Here's the drawing with two shaded views (mm, measured from the low corner). I have some questions. A direction names the side the tool comes from. Give positions to 0.01 mm unless a question says otherwise; leave off trailing zeros. Loops run counter-clockwise (first coordinate to the right, second up) from the corner with the lowest first, then second, coordinate; pieces in that order, holes last. Notation, with made-up numbers: M 25.25,-33 L 68.25,-33 A8 cw 68.25,-24 Z; hole C 24.25,6 d3. An arc over 180 degrees is marked long. Use a Markdown table: item, result. Add a question column.
1) Suppose I cut it at D-D on x = 7.5. List the corners of the cut face in (y, z) for me.
2) Suppose I cut it at A-A on y = 14.25. List the corners of the cut face in (x, z) for me (3 decimals).
3) Will these pins go through, and if not, where does the flat tip stop? pin 1 Ø16 at (y, z) = (14.25, 14.25) entering from +X; pin 2 Ø5 at (x, y) = (8.5, 10) entering from -Z; pin 3 Ø12.5 at (y, z) = (14.25, 14.25) entering from -X; pin 4 Ø3 at (x, z) = (1.5, 5.5) entering from +Y.
4) We'd pull the mould along Y, two halves only. Please class the marked faces 1, 2, 3 and 4: +Y half, -Y half, draft (parallel to the pull), parting line (faces both ways), or undercut.
5) Suppose I cut it at C-C on x = 1.5. List the corners of the cut face in (y, z) for me.
6) If I drill on line 1 along Y through (x, z) = (3.25, 14.25); line 2 along Z through (x, y) = (10.5, 14.25) (3 decimals); line 3 along Z through (x, y) = (8.25, 14.25), over which ranges is the centre line in solid material (lowest first)? Write a range as [from, to].
7) Which directions (+Z, -Z, +X, -X, +Y, -Y) give clear straight access to the entire face, cutting with the end or side of a thin tool? Please do the marked faces 5 and 6.
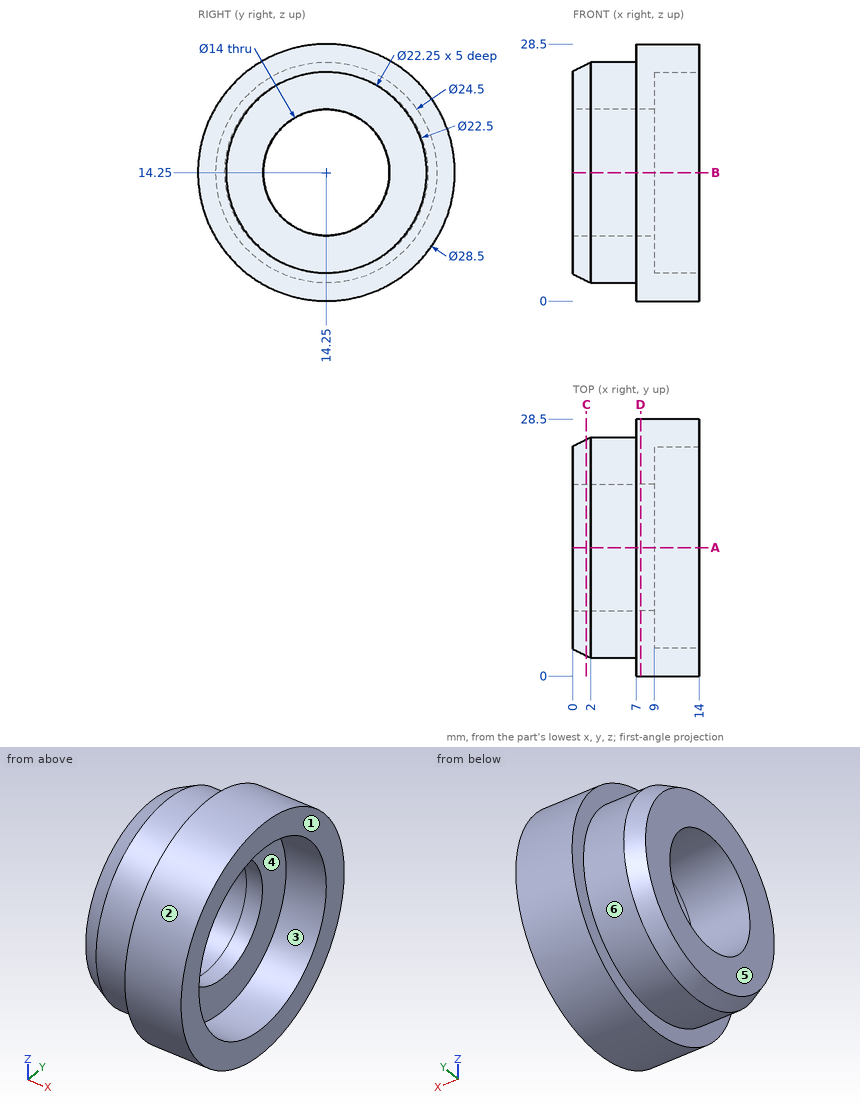
Answer block:
| question | item | result |
|---|---|---|
| 1 | outline | C 14.25,14.25 d28.5; hole C 14.25,14.25 d14 |
| 2 | outline | M 0,3 L 2,2 L 7,2 L 7,0 L 14,0 L 14,3.125 L 9,3.125 L 9,7.25 L 0,7.25 Z; M 0,21.25 L 9,21.25 L 9,25.375 L 14,25.375 L 14,28.5 L 7,28.5 L 7,26.5 L 2,26.5 L 0,25.5 Z |
| 3 | pin 1 | stops at x = 9 |
| 3 | pin 2 | stops at z = 0.11 |
| 3 | pin 3 | passes through |
| 3 | pin 4 | stops at y = 24.06 |
| 4 | face 1 | draft |
| 4 | face 2 | parting line |
| 4 | face 3 | undercut |
| 4 | face 4 | undercut |
| 5 | outline | C 14.25,14.25 d24; hole C 14.25,14.25 d14 |
| 6 | line 1 | y = [2, 7.25], [21.25, 26.5] |
| 6 | line 2 | z = [0, 3.125], [25.375, 28.5] |
| 6 | line 3 | z = [0, 7.25], [21.25, 28.5] |
| 7 | face 5 | +Z, -Z, -X, +Y, -Y |
| 7 | face 6 | -X |
